Can you work these out from the model? Positions are in its coordinate system, mm. Face numbers are marked on the shaded views. A direction names the side the tool comes from. Give positions to 0.01 mm unless a question says otherwise; leave off trailing zeros. Loops run counter-clockwise (first coordinate to the right, second up) from the corner with the lowest first, then second, coordinate; pieces in that order, holes last. Notation, with made-up numbers: (-15, 60.25) - (9, 60.25) arc R10 cw to (9, 79.25) - close; hole circle Ø7 at (48.25, 49). An arc over 180 degrees is marked (long way). Answer as a JSON object with one key per item and string values.
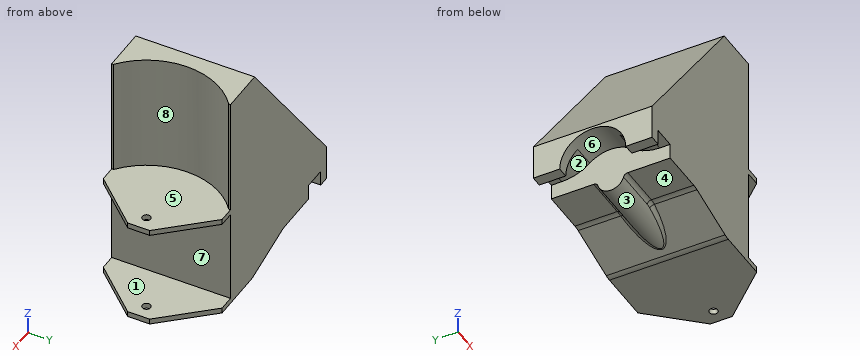
Solid Edge part; units mm, degrees
sketch "Sketch1" plane through (0, 0, 0) normal (0, -1, 0) x (1, 0, 0)
  line L0 (0, 0) -> (0, 51)
  line L1 (0, 51) -> (-10, 51)
  line L2 (-10, 51) -> (-40, 11.65)
  line L3 (-40, 3.65) -> (-40, 11.65)
  line L4 (-40, 3.65) -> (-22, 3.65)
  line L5 (-9, 0) -> (-22, 3.65)
  line L6 (0, 0) -> (-9, 0)
extrude "Protrusion1" add sketch "Sketch1" along normal mid plane 27
sketch "Sketch2" plane through (-5, 0, 51) normal (0, 0, 1) x (0, -1, 0)
  circle A0 centre (0, 15.25) radius 16.625
extrude "ExtrudedCutout_1" cut sketch "Sketch2" against normal blind 27
sketch "Sketch3" plane through (-20, -13.5, 25.5) normal (0, -1, 0) x (1, 0, 0)
  line L0 (-17.5, -21.85) -> (-12.5, -21.85)
  line L1 (-12.5, -21.85) -> (-12.5, -18.35)
  line L2 (-12.5, -18.35) -> (-17.5, -18.35)
  line L3 (-17.5, -18.35) -> (-17.5, -21.85)
extrude "Cutout1" cut sketch "Sketch3" against normal through all
sketch "Sketch4" plane through (-40, 0, 7.65) normal (-1, 0, 0) x (0, -1, 0)
  arc A0 (7.5, -4) -> (-7.5, -4) centre (0, -4) ccw
extrude "Cutout2" cut sketch "Sketch4" against normal up to surface (7.5 mm away) material side at (-40, 0, 11.1)
fillet "Round_1" radius 10 2 edges at (-35, -6.6332, 7.15) (-35, 6.6332, 7.15)
sketch "Sketch5" plane through (0, 0, 0) normal (0, 0, -1) x (-1, 0, 0)
  line L0 (0, 13.5) -> (0, -13.5)
  line L1 (0, -13.5) -> (-3.5, -13.5)
  line L2 (-3.5, -13.5) -> (-13.5, -2.5)
  line L3 (-13.5, -2.5) -> (-13.5, 2.5)
  line L4 (-13.5, 2.5) -> (-3.5, 13.5)
  line L5 (0, 13.5) -> (-3.5, 13.5)
  circle A0 centre (-10.25, 0) radius 0.95
extrude "ExtrudedProtrusion_2" add sketch "Sketch5" against normal blind 1.25
mirror "Mirror1" about plane through (2.25, 0, 12) normal (0, 0, -1) of "ExtrudedProtrusion_2"
fillet "Round_2" radius 5 2 edges at (-22, 0, 3.65) (-9, 0, 0)
sketch "Sketch6" plane through (-32.5, 0, 7.4) normal (-1, 0, 0) x (0, -1, 0)
  circle A0 centre (0, -3.75) radius 3
extrude "Protrusion3" add sketch "Sketch6" against normal up to vertex (22.837 mm away)
fillet "Round_3" radius 1 5 edges at (-27.5943, -3, 3.65) (-22.0064, -2.9996, 3.6032) (-11.3151, 0, 0.65) (-22.0064, 2.9996, 3.6032) (-27.5943, 3, 3.65)
properties material "Stainless Steel, 420"
1) I need wall thicknesses on L1, parallel to Z at x = 6, y = 6.25; L2, parallel to Z at x = -2, y = -2.5; L3, parallel to Y at x = 10.25, z = 0.6 (3 decimals). Which ranges of each line are inside material? Lowest first, please.
Check sheet entries:
{"L1": "0 to 1.25, 22.75 to 24", "L2": "0 to 24", "L3": "-6.075 to -0.95, 0.95 to 6.075"}
2) Imagine slicing it at C-C on y = -6. Write out the boundary of the cut face in (x, z), and give its area (3 significant figures).
Check sheet entries:
{"outline": "(-40, 8.15) - (-37.5, 8.15) - (-37.5, 8.57) - (-32.5, 8.57) - (-32.5, 3.65) - (-22.69, 3.65) arc R5 cw to (-21.34, 3.46) - (-9.66, 0.19) arc R5 ccw to (-8.31, 0) - (10.32, 0) - (10.32, 1.25) - (0, 1.25) - (0, 22.75) - (10.32, 22.75) - (10.32, 24) - (-5.25, 24) - (-5.25, 51) - (-10, 51) - (-40, 11.65) - close", "area": "1,210 mm2"}
3) Imagine slicing it at A-A on x = 10.25. Write out the boundary of the cut face in (y, z) (3 decimals).
Check sheet entries:
{"outline": "(-6.075, 0) - (-0.95, 0) - (-0.95, 1.25) - (-6.075, 1.25) - close; (-6.075, 22.75) - (-0.95, 22.75) - (-0.95, 24) - (-6.075, 24) - close; (0.95, 0) - (6.075, 0) - (6.075, 1.25) - (0.95, 1.25) - close; (0.95, 22.75) - (6.075, 22.75) - (6.075, 24) - (0.95, 24) - close"}
4) Imagine slicing it at D-D on x = -5.5. Write out the boundary of the cut face in (y, z), and give its area (3 significant figures).
Check sheet entries:
{"outline": "(-13.5, 0) - (13.5, 0) - (13.5, 51) - (5.32, 51) - (5.32, 24) - (-5.32, 24) - (-5.32, 51) - (-13.5, 51) - close", "area": "1,090 mm2"}
5) I'm going to push flat-ended pins straight in: P1, Ø6.5, axis at y = 11, z = 7, coming from the +X side; P2, Ø1.2, axis at x = -34, y = 13, coming from the -Z side; P3, Ø3, axis at x = -38.5, y = 9.5, coming from the -Z side; P4, Ø7, axis at x = 5, y = -2.5, coming from the -Z side. Where does each tip first touch, or does it pass through?
Check sheet entries:
{"P1": "x = 0", "P2": "z = 7.15", "P3": "z = 3.65", "P4": "z = 0"}
6) If we mould it in two halves opening along Z, with no side actions, what happens to the marked faces 6, 7 and 8? For each: released by +Z, released by -Z, zero draft, split by the parting line, or undercut.
Check sheet entries:
{"face 6": "released by -Z", "face 7": "undercut", "face 8": "zero draft"}
7) Which directions (+Z, -Z, +X, -X, +Y, -Y) give clear straight access to the entire face, cutting with the end or side of a thin tool? Please do the marked faces 1, 2, 3, 4 and 5.
Check sheet entries:
{"face 1": "+X, +Y, -Y", "face 2": "-Z", "face 3": "-Z, -X", "face 4": "-Z, -X, -Y", "face 5": "+Z, +X"}
8) Imagine slicing it at B-B on y = 0. Give the number of separate pieces and of enclosed holes in the cut face, and give its area (3 significant figures).
Check sheet entries:
{"separate pieces": "3", "enclosed holes": "0", "area": "1,210 mm2"}
